Work out the finished part from the listing and answer in its coordinate system (mm). Round coordinates to 2 decimals unless told otherwise and drop trailing zeros. Order: outer loops, then holes, each group sorted by start corner. A loop starts at its lowest first (then second) coordinate and runs counter-clockwise, first axis right, second up. Notation, with made-up numbers: M 54.5,50.25 L 90.5,50.25 A24 ccw 90.5,88.25 Z; hole C 61.25,-11.5 d11. An arc over 180 degrees is marked long. Return JSON: item names as keys, results as strings.
from build123d import *

# Parameters (mm, degrees)
SKETCH3_W           = 88
SKETCH3_H           = 30
BOSS_EXTRUDE1_DEPTH = 3.175
CUT_EXTRUDE1_REACH  = 5.175
SKETCH4_W           = 3.175
SKETCH4_H           = 7.825
SKETCH4_W_2         = 8
SKETCH4_H_2         = 3.175
SKETCH4_H_3         = 11
CUT_EXTRUDE2_REACH  = 5.175
SKETCH5_R           = 2


with BuildPart() as part:
    # Sketch3 → Boss-Extrude1 (new body)
    with BuildSketch(Plane(origin=(0, 0, 0), x_dir=(1, 0, 0), z_dir=(0, 1, 0))):
        with Locations((44, -15)):
            Rectangle(SKETCH3_W, SKETCH3_H)
    extrude(amount=BOSS_EXTRUDE1_DEPTH)

    # Sketch4 → Cut-Extrude1 (cut, up to next)
    with BuildSketch(Plane(origin=(0, 3.175, 0), x_dir=(1, 0, 0), z_dir=(0, 1, 0)), mode=Mode.PRIVATE) as cut_extrude1_sk1:
        with Locations((1.5875, -22.9125)):
            Rectangle(SKETCH4_W, SKETCH4_H)
    cut_extrude1_tool1 = extrude(cut_extrude1_sk1.sketch, amount=-CUT_EXTRUDE1_REACH, mode=Mode.PRIVATE) & part.part
    add(cut_extrude1_tool1.solids().sort_by_distance((1.5875, 3.175, 22.9125))[0], mode=Mode.SUBTRACT)
    # Sketch4 → Cut-Extrude1 (cut, up to next)
    with BuildSketch(Plane(origin=(0, 3.175, 0), x_dir=(1, 0, 0), z_dir=(0, 1, 0)), mode=Mode.PRIVATE) as cut_extrude1_sk2:
        Polygon((0, -30), (16, -30), (16, -26.825), (3.175, -26.825), (0, -26.825), align=None)
    cut_extrude1_tool2 = extrude(cut_extrude1_sk2.sketch, amount=-CUT_EXTRUDE1_REACH, mode=Mode.PRIVATE) & part.part
    add(cut_extrude1_tool2.solids().sort_by_distance((8, 3.175, 28.4125))[0], mode=Mode.SUBTRACT)
    # Sketch4 → Cut-Extrude1 (cut, up to next)
    with BuildSketch(Plane(origin=(0, 3.175, 0), x_dir=(1, 0, 0), z_dir=(0, 1, 0)), mode=Mode.PRIVATE) as cut_extrude1_sk3:
        with Locations((28, -28.4125)):
            Rectangle(SKETCH4_W_2, SKETCH4_H_2)
    cut_extrude1_tool3 = extrude(cut_extrude1_sk3.sketch, amount=-CUT_EXTRUDE1_REACH, mode=Mode.PRIVATE) & part.part
    add(cut_extrude1_tool3.solids().sort_by_distance((28, 3.175, 28.4125))[0], mode=Mode.SUBTRACT)
    # Sketch4 → Cut-Extrude1 (cut, up to next)
    with BuildSketch(Plane(origin=(0, 3.175, 0), x_dir=(1, 0, 0), z_dir=(0, 1, 0)), mode=Mode.PRIVATE) as cut_extrude1_sk4:
        with Locations((44, -28.4125)):
            Rectangle(SKETCH4_W_2, SKETCH4_H_2)
    cut_extrude1_tool4 = extrude(cut_extrude1_sk4.sketch, amount=-CUT_EXTRUDE1_REACH, mode=Mode.PRIVATE) & part.part
    add(cut_extrude1_tool4.solids().sort_by_distance((44, 3.175, 28.4125))[0], mode=Mode.SUBTRACT)
    # Sketch4 → Cut-Extrude1 (cut, up to next)
    with BuildSketch(Plane(origin=(0, 3.175, 0), x_dir=(1, 0, 0), z_dir=(0, 1, 0)), mode=Mode.PRIVATE) as cut_extrude1_sk5:
        with Locations((60, -28.4125)):
            Rectangle(SKETCH4_W_2, SKETCH4_H_2)
    cut_extrude1_tool5 = extrude(cut_extrude1_sk5.sketch, amount=-CUT_EXTRUDE1_REACH, mode=Mode.PRIVATE) & part.part
    add(cut_extrude1_tool5.solids().sort_by_distance((60, 3.175, 28.4125))[0], mode=Mode.SUBTRACT)
    # Sketch4 → Cut-Extrude1 (cut, up to next)
    with BuildSketch(Plane(origin=(0, 3.175, 0), x_dir=(1, 0, 0), z_dir=(0, 1, 0)), mode=Mode.PRIVATE) as cut_extrude1_sk6:
        with Locations((86.4125, -22.9125)):
            Rectangle(SKETCH4_W, SKETCH4_H)
    cut_extrude1_tool6 = extrude(cut_extrude1_sk6.sketch, amount=-CUT_EXTRUDE1_REACH, mode=Mode.PRIVATE) & part.part
    add(cut_extrude1_tool6.solids().sort_by_distance((86.4125, 3.175, 22.9125))[0], mode=Mode.SUBTRACT)
    # Sketch4 → Cut-Extrude1 (cut, up to next)
    with BuildSketch(Plane(origin=(0, 3.175, 0), x_dir=(1, 0, 0), z_dir=(0, 1, 0)), mode=Mode.PRIVATE) as cut_extrude1_sk7:
        with Locations((86.4125, -5.5)):
            Rectangle(SKETCH4_W, SKETCH4_H_3)
    cut_extrude1_tool7 = extrude(cut_extrude1_sk7.sketch, amount=-CUT_EXTRUDE1_REACH, mode=Mode.PRIVATE) & part.part
    add(cut_extrude1_tool7.solids().sort_by_distance((86.4125, 3.175, 5.5))[0], mode=Mode.SUBTRACT)
    # Sketch4 → Cut-Extrude1 (cut, up to next)
    with BuildSketch(Plane(origin=(0, 3.175, 0), x_dir=(1, 0, 0), z_dir=(0, 1, 0)), mode=Mode.PRIVATE) as cut_extrude1_sk8:
        Polygon((72, -26.825), (72, -30), (88, -30), (88, -26.825), (84.825, -26.825), align=None)
    cut_extrude1_tool8 = extrude(cut_extrude1_sk8.sketch, amount=-CUT_EXTRUDE1_REACH, mode=Mode.PRIVATE) & part.part
    add(cut_extrude1_tool8.solids().sort_by_distance((80, 3.175, 28.4125))[0], mode=Mode.SUBTRACT)
    # Sketch4 → Cut-Extrude1 (cut, up to next)
    with BuildSketch(Plane(origin=(0, 3.175, 0), x_dir=(1, 0, 0), z_dir=(0, 1, 0)), mode=Mode.PRIVATE) as cut_extrude1_sk9:
        with Locations((1.5875, -5.5)):
            Rectangle(SKETCH4_W, SKETCH4_H_3)
    cut_extrude1_tool9 = extrude(cut_extrude1_sk9.sketch, amount=-CUT_EXTRUDE1_REACH, mode=Mode.PRIVATE) & part.part
    add(cut_extrude1_tool9.solids().sort_by_distance((1.5875, 3.175, 5.5))[0], mode=Mode.SUBTRACT)

    # Sketch5 → Cut-Extrude2 (cut, up to next)
    with BuildSketch(Plane(origin=(0, 3.175, 0), x_dir=(1, 0, 0), z_dir=(0, 1, 0)), mode=Mode.PRIVATE) as cut_extrude2_sk1:
        with Locations((44, -8.9125)):
            Circle(SKETCH5_R)
    cut_extrude2_tool1 = extrude(cut_extrude2_sk1.sketch, amount=-CUT_EXTRUDE2_REACH, mode=Mode.PRIVATE) & part.part
    add(cut_extrude2_tool1.solids().sort_by_distance((44, 3.175, 8.9125))[0], mode=Mode.SUBTRACT)
    # Sketch5 → Cut-Extrude2 (cut, up to next)
    with BuildSketch(Plane(origin=(0, 3.175, 0), x_dir=(1, 0, 0), z_dir=(0, 1, 0)), mode=Mode.PRIVATE) as cut_extrude2_sk2:
        with Locations((9, -8.9125)):
            Circle(SKETCH5_R)
    cut_extrude2_tool2 = extrude(cut_extrude2_sk2.sketch, amount=-CUT_EXTRUDE2_REACH, mode=Mode.PRIVATE) & part.part
    add(cut_extrude2_tool2.solids().sort_by_distance((9, 3.175, 8.9125))[0], mode=Mode.SUBTRACT)
    # Sketch5 → Cut-Extrude2 (cut, up to next)
    with BuildSketch(Plane(origin=(0, 3.175, 0), x_dir=(1, 0, 0), z_dir=(0, 1, 0)), mode=Mode.PRIVATE) as cut_extrude2_sk3:
        with Locations((79, -8.9125)):
            Circle(SKETCH5_R)
    cut_extrude2_tool3 = extrude(cut_extrude2_sk3.sketch, amount=-CUT_EXTRUDE2_REACH, mode=Mode.PRIVATE) & part.part
    add(cut_extrude2_tool3.solids().sort_by_distance((79, 3.175, 8.9125))[0], mode=Mode.SUBTRACT)
    # Sketch5 → Cut-Extrude2 (cut, up to next)
    with BuildSketch(Plane(origin=(0, 3.175, 0), x_dir=(1, 0, 0), z_dir=(0, 1, 0)), mode=Mode.PRIVATE) as cut_extrude2_sk4:
        with BuildLine():
            Line((75.5, -8.9125), (75.5, 0))
            Line((75.5, 0), (47.5, 0))
            Line((47.5, 0), (47.5, -8.9125))
            ThreePointArc((47.5, -8.9125), (61.5, -22.9125), (75.5, -8.9125))
        make_face()
    cut_extrude2_tool4 = extrude(cut_extrude2_sk4.sketch, amount=-CUT_EXTRUDE2_REACH, mode=Mode.PRIVATE) & part.part
    add(cut_extrude2_tool4.solids().sort_by_distance((61.5, 3.175, 10.199265))[0], mode=Mode.SUBTRACT)
    # Sketch5 → Cut-Extrude2 (cut, up to next)
    with BuildSketch(Plane(origin=(0, 3.175, 0), x_dir=(1, 0, 0), z_dir=(0, 1, 0)), mode=Mode.PRIVATE) as cut_extrude2_sk5:
        with BuildLine():
            Line((12.5, -8.9125), (12.5, 0))
            Line((12.5, 0), (40.5, 0))
            Line((40.5, 0), (40.5, -8.9125))
            ThreePointArc((40.5, -8.9125), (26.5, -22.9125), (12.5, -8.9125))
        make_face()
    cut_extrude2_tool5 = extrude(cut_extrude2_sk5.sketch, amount=-CUT_EXTRUDE2_REACH, mode=Mode.PRIVATE) & part.part
    add(cut_extrude2_tool5.solids().sort_by_distance((26.5, 3.175, 10.199265))[0], mode=Mode.SUBTRACT)


solid = part.part
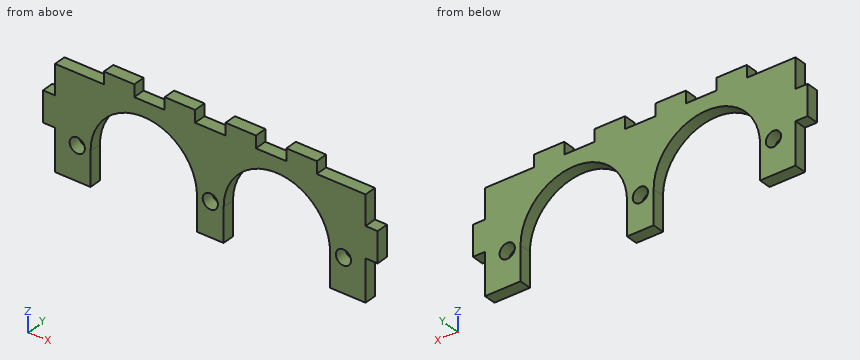
Item 1: Consider line 1 along X through (y, z) = (2.75, 4.75) (3 decimals); line 2 along X through (y, z) = (1.2, 28.5); line 3 along Z through (x, y) = (9, 1.65) (1 decimal). Determine where each line is inside the solid, lowest interval first. Write a range as [from, to].
Output:
{"line 1": "x = [3.175, 12.5], [40.5, 47.5], [75.5, 84.825]", "line 2": "x = [16, 24], [32, 40], [48, 56], [64, 72]", "line 3": "z = [0, 6.9], [10.9, 26.8]"}
Item 2: Each of these flat-tipped pins is pushed along its axis until it touches: pin 1 (1.6 mm diameter, centred on y = 1.5, z = 4, fed in from -X) (3 decimals); pin 2 (1.6 mm diameter, centred on x = 43, y = 2, fed in from +Z) (3 decimals); pin 3 (1.6 mm diameter, centred on y = 2, z = 6, fed in from +X) (3 decimals). Where does it stop, or does it pass through?
Output:
{"pin 1": "stops at x = 3.175", "pin 2": "stops at z = 26.825", "pin 3": "stops at x = 84.825"}
Item 3: Find section A-A (x = 44). Determine the outline of the cut face in (y, z) (1 decimal).
Output:
{"outline": "M 0,0 L 3.2,0 L 3.2,6.9 L 0,6.9 Z; M 0,10.9 L 3.2,10.9 L 3.2,26.8 L 0,26.8 Z"}
Item 4: Find section D-D (y = 1.65). State how many separate pieces and enclosed holes the cut face has, plus the area to 3 significant figures.
Output:
{"separate pieces": "1", "enclosed holes": "3", "area": "1,190 mm^2"}
Item 5: Find section C-C (x = 10). Determine the outline of the cut face in (y, z) (3 decimals).
Output:
{"outline": "M 0,0 L 3.175,0 L 3.175,7.18 L 0,7.18 Z; M 0,10.645 L 3.175,10.645 L 3.175,26.825 L 0,26.825 Z"}
Item 6: Find section B-B (z = 24.25). Determine the outline of the cut face in (x, y) (3 decimals), plus the area to 3 significant figures.
Output:
{"outline": "M 3.175,0 L 84.825,0 L 84.825,3.175 L 3.175,3.175 Z", "area": "259 mm^2"}
